```python
from build123d import *

# Parameters (mm, degrees)
BOSS_EXTRUDE1_DEPTH     = 3.175
SKETCH2_R               = 19.9
CUT_EXTRUDE1_DEPTH      = 140.49939292
ESQUISSE2_R             = 1.5
ENL_V_MAT_EXTRU_1_DEPTH = 140.49939292
SKETCH5_R               = 1.625
CUT_EXTRUDE3_DEPTH      = 140.49939292
CUT_EXTRUDE4_DEPTH      = 140.49939292


with BuildPart() as part:
    # Sketch1 → Boss-Extrude1 (new body)
    with BuildSketch(Plane(origin=(0, 0, 0), x_dir=(1, 0, 0), z_dir=(0, 1, 0))):
        with BuildLine():
            Line((-27.5, -100), (-34.975254116, 98.684097441))
            ThreePointArc((-34.975254116, 98.684097441), (0, 135), (34.975254116, 98.684097441))
            Line((34.975254116, 98.684097441), (27.5, -100))
            ThreePointArc((27.5, -100), (0, -127.5), (-27.5, -100))
        make_face()
    extrude(amount=BOSS_EXTRUDE1_DEPTH)

    # Sketch2 → Cut-Extrude1 (cut, through all)
    with BuildSketch(Plane(origin=(0, 3.175, 0), x_dir=(1, 0, 0), z_dir=(0, 1, 0))):
        with Locations(Location((0, -100, 0), (0, 0, 270))):
            Circle(SKETCH2_R)
        with Locations(Location((0, 100, 0), (0, 0, 270))):
            Circle(SKETCH2_R)
    extrude(amount=-CUT_EXTRUDE1_DEPTH, mode=Mode.SUBTRACT)

    # Esquisse2 → Enlèv. mat.-Extru.1 (cut, through all)
    with BuildSketch(Plane(origin=(0, 3.175, 0), x_dir=(1, 0, 0), z_dir=(0, 1, 0))):
        with Locations(Location((19.339370465, 80.660629535, 0), (0, 0, 270))):
            Circle(ESQUISSE2_R)
        with Locations(Location((19.339370465, 119.339370465, 0), (0, 0, 270))):
            Circle(ESQUISSE2_R)
        with Locations(Location((-19.339370465, 119.339370465, 0), (0, 0, 270))):
            Circle(ESQUISSE2_R)
        with Locations(Location((-19.339370465, 80.660629535, 0), (0, 0, 270))):
            Circle(ESQUISSE2_R)
    extrude(amount=-ENL_V_MAT_EXTRU_1_DEPTH, mode=Mode.SUBTRACT)

    # Sketch5 → Cut-Extrude3 (cut, through all)
    with BuildSketch(Plane(origin=(0, 3.175, 0), x_dir=(1, 0, 0), z_dir=(0, 1, 0))):
        with Locations(Location((-27.331724457, 46.340455159, 0), (0, 0, 270))):
            Circle(SKETCH5_R)
        with Locations(Location((-26.316599626, 19.359544841, 0), (0, 0, 270))):
            Circle(SKETCH5_R)
        with Locations(Location((26.316599626, 19.359544841, 0), (0, 0, 270))):
            Circle(SKETCH5_R)
        with Locations(Location((27.331724457, 46.340455159, 0), (0, 0, 270))):
            Circle(SKETCH5_R)
        Polygon((-21.15, 49.828069991), (-16.978069991, 54), (16.978069991, 54), (21.15, 49.828069991), (21.15, 15.871930009), (16.978069991, 11.7), (-16.978069991, 11.7), (-21.15, 15.871930009), align=None)
    extrude(amount=-CUT_EXTRUDE3_DEPTH, mode=Mode.SUBTRACT)

    # Sketch7 → Cut-Extrude4 (cut, through all)
    with BuildSketch(Plane(origin=(0, 3.175, 0), x_dir=(1, 0, 0), z_dir=(0, 1, 0))):
        with BuildLine():
            Line((17.5, -43.3), (17.5, -3.3))
            ThreePointArc((17.5, -3.3), (15, -0.8), (12.5, -3.3))
            Line((12.5, -3.3), (12.5, -43.3))
            ThreePointArc((12.5, -43.3), (15, -45.8), (17.5, -43.3))
        make_face()
        with BuildLine():
            Line((-12.5, -43.3), (-12.5, -3.3))
            ThreePointArc((-12.5, -3.3), (-15, -0.8), (-17.5, -3.3))
            Line((-17.5, -3.3), (-17.5, -43.3))
            ThreePointArc((-17.5, -43.3), (-15, -45.8), (-12.5, -43.3))
        make_face()
    extrude(amount=-CUT_EXTRUDE4_DEPTH, mode=Mode.SUBTRACT)


solid = part.part
```
Input: part model. Units: mm. Frame: model coordinates. A direction names the side the tool comes from. Give positions to 0.01 mm unless a question says otherwise; leave off trailing zeros. Loops run counter-clockwise (first coordinate to the right, second up) from the corner with the lowest first, then second, coordinate; pieces in that order, holes last.
1) Reachability of faces 5 (the flat face through (-19.093, 1.61, -51.885)), 6 (the flat face through (-31.185, 1.565, 2.049)) from +Z, -Z, +X, -X, +Y, -Y: full face, straight path, thin tool, end or side. Return the list, or none.
A:
face 5: +Y, -Y
face 6: +Z, -X, +Y, -Y
2) Contact query for flat-ended pins moving along their axis: pin 1 (3 mm diameter, centred on x = -27.33, z = -46.34, fed in from -Y); pin 2 (1 mm diameter, centred on y = 2, z = 22.5, fed in from -X); pin 3 (4 mm diameter, centred on x = 16, z = 22, fed in from +Y) (3 decimals); pin 4 (1.6 mm diameter, centred on y = 2, z = 26.5, fed in from -X). Output: stop coordinate, or through.
A:
pin 1: passes through
pin 2: stops at x = -30.43
pin 3: stops at y = 3.175
pin 4: stops at x = -30.3
3) Section query C-C on y = 0.8. Count the separate pieces of the cut face and the enclosed holes in it, and give its area (3 significant figures).
A:
separate pieces: 1
enclosed holes: 13
area: 10,900 mm2
4) Section query A-A on x = 0. Return the cut outline in (y, z) (3 decimals).
A:
outline: (0, -135) - (3.175, -135) - (3.175, -119.9) - (0, -119.9) - close; (0, -80.1) - (3.175, -80.1) - (3.175, -54) - (0, -54) - close; (0, -11.7) - (3.175, -11.7) - (3.175, 80.1) - (0, 80.1) - close; (0, 119.9) - (3.175, 119.9) - (3.175, 127.5) - (0, 127.5) - close
5) Mould query, pull axis X, two halves, no side actions, for faces 1 (the flat face through (0, 3.175, -6)), 2 (the flat face through (19.093, 1.61, -13.815)), 3 (the cylindrical face through (0.605, 1.565, 127.493)), 4 (the flat face through (31.29, 1.57, -0.73)). Classes: released by +X, released by -X, zero draft, split by the parting line, or undercut.
A:
face 1: zero draft
face 2: undercut
face 3: split by the parting line
face 4: released by +X
6) Section query B-B on z = -40. Return the cut outline in (x, y) (3 decimals), and give its area (3 significant figures).
A:
outline: (-32.767, 0) - (-21.15, 0) - (-21.15, 3.175) - (-32.767, 3.175) - close; (21.15, 0) - (32.767, 0) - (32.767, 3.175) - (21.15, 3.175) - close
area: 73.8 mm2
7) Section query D-D on x = 10. Return the cut outline in (y, z) (3 decimals), and give its area (3 significant figures).
A:
outline: (0, -133.541) - (3.175, -133.541) - (3.175, -117.205) - (0, -117.205) - close; (0, -82.795) - (3.175, -82.795) - (3.175, -54) - (0, -54) - close; (0, -11.7) - (3.175, -11.7) - (3.175, 82.795) - (0, 82.795) - close; (0, 117.205) - (3.175, 117.205) - (3.175, 125.617) - (0, 125.617) - close
area: 470 mm2
8) Line query: L1, parallel to X at y = 0.5, z = 28; L2, parallel to Z at x = -4.5, y = 2.6; L3, parallel to X at y = 0.75, z = 99. Output: solid intervals per line, ascending.
A:
L1: x = -30.21 to -17.5, -12.5 to 12.5, 17.5 to 30.21
L2: z = -134.71 to -119.38, -80.62 to -54, -11.7 to 80.62, 119.38 to 127.13
L3: x = -27.54 to -19.87, 19.87 to 27.54
